```python
from build123d import *

# Parameters (mm, degrees)
SKETCH1_W               = 4
SKETCH1_H               = 2
BOSS_EXTRUDE1_DEPTH     = 12
BOSS_EXTRUDE2_DEPTH     = 1.5
CUT_EXTRUDE2_DEPTH      = 16.859104004
CUT_EXTRUDE2_DEPTH_BACK = 16.859104004


with BuildPart() as part:
    # Sketch1 → Boss-Extrude1 (new body)
    with BuildSketch(Plane.XY):
        with Locations((0, 1)):
            Rectangle(SKETCH1_W, SKETCH1_H)
    extrude(amount=BOSS_EXTRUDE1_DEPTH)

    # Sketch2 → Boss-Extrude2 (add)
    with BuildSketch(Plane(origin=(0, 0, 0), x_dir=(-1, 0, 0), z_dir=(0, 0, -1))):
        with BuildLine():
            Line((-2.6, 6.516547752), (-2.6, 8.116577001))
            ThreePointArc((-2.6, 8.116577001), (-3.392405194, 9.094791904), (-4.513808793, 8.522721667))
            ThreePointArc((-4.513808793, 8.522721667), (0, 1.576992752), (4.513808793, 8.522721667))
            ThreePointArc((4.513808793, 8.522721667), (3.392405194, 9.094791904), (2.6, 8.116577001))
            Line((2.6, 8.116577001), (2.6, 6.516547752))
            ThreePointArc((2.6, 6.516547752), (0, 3.916547752), (-2.6, 6.516547752))
        make_face()
    extrude(amount=-BOSS_EXTRUDE2_DEPTH)

    # Sketch3 → Cut-Extrude2 (cut, two sides: drawn at the far end of the back side and taken through both)
    with BuildSketch(Plane(origin=(0, 0, 0), x_dir=(0, 0, -1), z_dir=(1, 0, 0)).offset(-CUT_EXTRUDE2_DEPTH_BACK)):
        Polygon((-0.13532, 9.116577001), (-1.5, 6.3), (-1.5, 9.116577001), align=None)
    extrude(amount=CUT_EXTRUDE2_DEPTH + CUT_EXTRUDE2_DEPTH_BACK, mode=Mode.SUBTRACT)


solid = part.part
```
Design review of the part built by this model. Coordinates are the model's own, in mm. A direction names the side the tool comes from. Coordinates: 2 decimals unless noted, no trailing zeros. Write each loop counter-clockwise with the first axis right and the second up, starting at its lowest first coordinate (ties: lowest second). Pieces come first, ordered by that corner, then holes.
1) Add section C-C (x = 0). Write out the cut boundary in (y, z).
2) Add section A-A (y = 5.5). Write out the cut boundary in (x, z), plus the area to 3 significant figures.
3) Mouldability with a two-part tool opening along X and no side actions: class faces 4 (the cylindrical face through (4.63, 4.79, 0.74)), 5 (the flat face through (0.1, 3.6, 0)), 6 (the cylindrical face through (-0.057, 3.917, 0.74)) as +X half, -X half, draft (parallel to the pull), parting line (faces both ways), or undercut.
4) To check wall thickness, follow L1, parallel to X at y = 1.5, z = 2.5; L2, parallel to Y at x = -1.5, z = 11.5; L3, parallel to Z at x = -2.5, y = 2.75. State the ranges of each line that lie inside material, in increasing order.
5) Add section D-D (y = 6.75). Write out the cut boundary in (x, z).
6) Add section B-B (z = 4.5). Write out the cut boundary in (x, y), plus the area to 3 significant figures.
7) Machinability: for faces 1 (the flat face through (-2.6, 7.1, 0.5)), 2 (the flat face through (0.1, 3.7, 1.5)), 3 (the flat face through (0, 1, 12)), which of the approach directions +Z, -Z, +X, -X, +Y, -Y give a long, thin tool a straight path to every point of the face, cutting with its end or side? Answer none if there is none.
8) Insertion check: pin 1 (1.6 mm diameter, centred on y = 1, z = 5, fed in from -X); pin 2 (1.5 mm diameter, centred on y = 7.5, z = 0.5, fed in from +X); pin 3 (3 mm diameter, centred on x = 0.5, z = 5.5, fed in from +Y). Each pin has a flat end and moves straight along its axis. Give the tip position at first contact, or say it passes through.
Check result:
1. outline: (0, 0) - (3.92, 0) - (3.92, 1.5) - (2, 1.5) - (2, 12) - (0, 12) - close
2. outline: (-4.83, 0) - (-2.39, 0) - (-2.39, 1.5) - (-4.83, 1.5) - close; (2.39, 0) - (4.83, 0) - (4.83, 1.5) - (2.39, 1.5) - close
2. area: 7.32 mm2
3. face 4: +X half
3. face 5: draft
3. face 6: undercut
4. L1: x = -2 to 2
4. L2: y = 0 to 2
4. L3: z = 0 to 1.5
5. outline: (-4.93, 0) - (-2.6, 0) - (-2.6, 1.28) - (-4.93, 1.28) - close; (2.6, 0) - (4.93, 0) - (4.93, 1.28) - (2.6, 1.28) - close
6. outline: (-2, 0) - (2, 0) - (2, 2) - (-2, 2) - close
6. area: 8.00 mm2
7. face 1: +Z, -Z, +Y
7. face 2: +Z, +X, -X, +Y
7. face 3: +Z, +X, -X, +Y, -Y
8. pin 1: stops at x = -2
8. pin 2: stops at x = 4.93
8. pin 3: stops at y = 2
